```python
from build123d import *

# Parameters (mm, degrees)
F1_DEPTH = 10
F2_R     = 10
F3_R     = 4
F4_DEPTH = 10


with BuildPart() as f1:
    # F0 (on Top) → F1 (new body)
    with BuildSketch(Plane.XY):
        with BuildLine():
            ThreePointArc((5.9699246226, 59.4), (5.9924764387, 59.6996233496), (6, 60))
            ThreePointArc((6, 60), (5.9924764387, 60.3003766504), (5.9699246226, 60.6))
            ThreePointArc((5.9699246226, 60.6), (-6, 60), (5.9699246226, 59.4))
        make_face()
        with BuildLine():
            ThreePointArc((5.9699246226, 60.6), (5.9924764387, 60.3003766504), (6, 60))
            ThreePointArc((6, 60), (5.9924764387, 59.6996233496), (5.9699246226, 59.4))
            ThreePointArc((5.9699246226, 59.4), (35.3699246226, 30), (5.9699246226, 0.6))
            ThreePointArc((5.9699246226, 0.6), (5.9924764387, 0.3003766504), (6, 0))
            ThreePointArc((6, 0), (5.9924764387, -0.3003766504), (5.9699246226, -0.6))
            ThreePointArc((5.9699246226, -0.6), (36.5699246226, 30), (5.9699246226, 60.6))
        make_face()
        with BuildLine():
            ThreePointArc((-5.9699246226, -0.6), (0, -6), (5.9699246226, -0.6))
            ThreePointArc((5.9699246226, -0.6), (5.9924764387, -0.3003766504), (6, 0))
            ThreePointArc((6, 0), (5.9924764387, 0.3003766504), (5.9699246226, 0.6))
            ThreePointArc((5.9699246226, 0.6), (0, 6), (-5.9699246226, 0.6))
            ThreePointArc((-5.9699246226, 0.6), (-6, 0), (-5.9699246226, -0.6))
        make_face()
        with BuildLine():
            ThreePointArc((-5.9699246226, -59.4), (-35.3699246226, -30), (-5.9699246226, -0.6))
            ThreePointArc((-5.9699246226, -0.6), (-6, 0), (-5.9699246226, 0.6))
            ThreePointArc((-5.9699246226, 0.6), (-36.5699246226, -30), (-5.9699246226, -60.6))
            ThreePointArc((-5.9699246226, -60.6), (-6, -60), (-5.9699246226, -59.4))
        make_face()
        with BuildLine():
            ThreePointArc((6, -60), (0.3003766504, -54.0075235613), (-5.9699246226, -59.4))
            ThreePointArc((-5.9699246226, -59.4), (-6, -60), (-5.9699246226, -60.6))
            ThreePointArc((-5.9699246226, -60.6), (0.3003766504, -65.9924764387), (6, -60))
        make_face()
    extrude(amount=F1_DEPTH)

    # F2
    f2_edges = [f1.edges().sort_by_distance(p)[0] for p in [
        (5.969925, -0.6, 5),
        (5.969925, 59.4, 5),
        (5.969925, 0.6, 5),
        (5.969925, 60.6, 5),
        (-5.969925, -60.6, 5),
        (-5.969925, -0.6, 5),
        (-5.969925, -59.4, 5),
        (-5.969925, 0.6, 5),
    ]]
    fillet(f2_edges, radius=F2_R)

    # F3 (on face) → F4 (cut, through all)
    with BuildSketch(Plane.XY.offset(10)):
        Circle(F3_R)
        with Locations((0, 60)):
            Circle(F3_R)
        with Locations((0, -60)):
            Circle(F3_R)
    extrude(amount=-F4_DEPTH, mode=Mode.SUBTRACT)


solid = f1.part
```
Read the model definition and answer for the solid it produces. Units are mm, in the model's axes. A direction names the side the tool comes from. Give positions to 0.01 mm unless a question says otherwise; leave off trailing zeros. Write each loop counter-clockwise with the first axis right and the second up, starting at its lowest first coordinate (ties: lowest second). Pieces come first, ordered by that corner, then holes. Notation, with made-up numbers: M 0.5,68.25 L 40.5,68.25 A25 cw 40.5,95.25 Z; hole C -27,71 d2. An arc over 180 degrees is marked long. Put each result on its own line as item: value. Start each with the question number.
1. For a pull along X with two mould halves and no side action, classify faces 3 (the cylindrical face through (36.564, 29.395, 4.93)), 4 (the cylindrical face through (-36.564, -29.395, 4.93)), 5 (the cylindrical face through (0, -6, 5)), 6 (the flat face through (0, 5, 10)) as released by +X, released by -X, zero draft, split by the parting line, or undercut.
2. The part is cut by section C-C, the plane y = 18.5. Give the vertices of the cut face in (x, z).
3. The part is cut by section A-A, the plane x = 0. Give the vertices of the cut face in (y, z), and give its area (3 significant figures).
4. Consider line 1 along Y through (x, z) = (0, 5); line 2 along Y through (x, z) = (5, 1.5); line 3 along X through (y, z) = (30, 9.75). Determine where each line is inside the solid, lowest interval first.
5. Each of these flat-tipped pins is pushed along its axis until it touches: pin 1 Ø6 at (y, z) = (11, 4) entering from -X; pin 2 Ø1.5 at (y, z) = (-9.5, 3) entering from +X; pin 3 Ø6 at (y, z) = (-21, 7) entering from -X. Where does it stop, or does it pass through?
6. The part is cut by section D-D, the plane y = -30.5. Give the vertices of the cut face in (x, z), and give its area (3 significant figures).
7. The part is cut by section B-B, the plane z = 2.5. Give the number of separate pieces and of enclosed holes in the cut face, and give its area (3 significant figures).
8. Which of the six approach directions +Z, -Z, +X, -X, +Y, -Y give full straight-line access (tool end or side, diameter ignored) to faces 1 (the cylindrical face through (-35.365, -30.532, 4.93)), 2 (the flat face through (0, 5, 0))?
Final values:
1. face 3: released by +X
1. face 4: released by -X
1. face 5: undercut
1. face 6: zero draft
2. outline: M 33.03,0 L 34.33,0 L 34.33,10 L 33.03,10 Z
3. outline: M -66,0 L -64,0 L -64,10 L -66,10 Z; M -56,0 L -54,0 L -54,10 L -56,10 Z; M -6,0 L -4,0 L -4,10 L -6,10 Z; M 4,0 L 6,0 L 6,10 L 4,10 Z; M 54,0 L 56,0 L 56,10 L 54,10 Z; M 64,0 L 66,0 L 66,10 L 64,10 Z
3. area: 120 mm²
4. line 1: y = -66 to -64, -56 to -54, -6 to -4, 4 to 6, 54 to 56, 64 to 66
4. line 2: y = -63.32 to -56.68, -3.38 to 3.56, 56.44 to 63.38
4. line 3: x = 35.37 to 36.57
5. pin 1: stops at x = 25.47
5. pin 2: stops at x = -26.29
5. pin 3: stops at x = -35.98
6. outline: M -36.57,0 L -35.37,0 L -35.37,10 L -36.57,10 Z
6. area: 12.0 mm²
7. separate pieces: 1
7. enclosed holes: 3
7. area: 456 mm²
8. face 1: +Z, -Z
8. face 2: -Z, +X, -X, +Y, -Y
